Part model, mm, in its own coordinate system. A direction names the side the tool comes from. Coordinates: 2 decimals unless noted, no trailing zeros. Loops run counter-clockwise (first coordinate to the right, second up) from the corner with the lowest first, then second, coordinate; pieces in that order, holes last. Notation, with made-up numbers: (-10.75, 77) - (-0.75, 77) arc R35 ccw to (-0.75, 111) - close; hole circle Ø8 at (-35, 6). An arc over 180 degrees is marked (long way). Answer as CSV lines item,"result".
from build123d import *

# Parameters (mm, degrees)
F0_W          = 200
F0_H          = 200
F1_DEPTH      = 100
F1_DEPTH_BACK = 100
F2_R          = 12.7
F3_R          = 25
F4_DEPTH      = 12.7
F5_R          = 25
F6_DEPTH      = 12.7
F7_R          = 25
F9_DEPTH      = 12.7
F10_R         = 25
F11_DEPTH     = 12.7
F12_R         = 25
F13_DEPTH     = 12.7
F14_R         = 25
F15_DEPTH     = 12.7


with BuildPart() as f1:
    # F0 (on Top) → F1 (new body, two sides)
    with BuildSketch(Plane.XY) as f1_sk:
        Rectangle(F0_W, F0_H)
    extrude(amount=F1_DEPTH)
    extrude(f1_sk.sketch, amount=-F1_DEPTH_BACK)

    # F2
    f2_edges = [f1.edges().sort_by_distance(p)[0] for p in [
        (100, 0, 100),
        (0, 100, 100),
        (-100, 0, 100),
        (0, -100, 100),
        (-100, -100, 0),
        (-100, 0, -100),
        (-100, 100, 0),
        (100, 0, -100),
        (0, 100, -100),
        (0, -100, -100),
        (100, 100, 0),
        (100, -100, 0),
    ]]
    fillet(f2_edges, radius=F2_R)

    # F3 (on face) → F4 (cut)
    with BuildSketch(Plane.XZ.offset(100)):
        Circle(F3_R)
    extrude(amount=-F4_DEPTH, mode=Mode.SUBTRACT)

    # F5 (on face) → F6 (cut)
    with BuildSketch(Plane(origin=(0, 100, 0), x_dir=(-1, 0, 0), z_dir=(0, 1, 0))):
        with Locations((-49.8331896961, 49.8331896961)):
            Circle(F5_R)
        with Locations((3.5068103039, 49.8331896961)):
            Circle(F5_R)
        with Locations((56.8468103039, 49.8331896961)):
            Circle(F5_R)
        with Locations((-49.8331896961, -49.2268103039)):
            Circle(F5_R)
        with Locations((3.5068103039, -49.2268103039)):
            Circle(F5_R)
        with Locations((56.8468103039, -49.2268103039)):
            Circle(F5_R)
    extrude(amount=-F6_DEPTH, mode=Mode.SUBTRACT)

    # F7 (on face) → F9 (cut)
    with BuildSketch(Plane(origin=(-100, 0, 0), x_dir=(0, -1, 0), z_dir=(-1, 0, 0))):
        with Locations((-43.65, 43.65)):
            Circle(F7_R)
        with BuildLine():
            ThreePointArc((24.561363538, -59.7938520193), (52.2460481749, -67.1256886113), (68.65, -43.65))
            ThreePointArc((68.65, -43.65), (67.1342312954, -35.077317779), (62.770729563, -27.5441718319))
            ThreePointArc((62.770729563, -27.5441718319), (27.5572450229, -24.5833313789), (24.561363538, -59.7938520193))
        make_face()
        with BuildLine():
            ThreePointArc((62.770729563, -27.5441718319), (67.1342312954, -35.077317779), (68.65, -43.65))
            ThreePointArc((68.65, -43.65), (52.2460481749, -67.1256886113), (24.561363538, -59.7938520193))
            ThreePointArc((24.561363538, -59.7938520193), (52.254775322, -67.1722551466), (68.6820931009, -43.6880238512))
            ThreePointArc((68.6820931009, -43.6880238512), (67.1577817122, -35.0919756763), (62.770729563, -27.5441718319))
        make_face()
        with BuildLine():
            ThreePointArc((24.561363538, -59.7938520193), (27.5572450229, -24.5833313789), (62.770729563, -27.5441718319))
            ThreePointArc((62.770729563, -27.5441718319), (27.525151922, -24.5453075277), (24.561363538, -59.7938520193))
        make_face()
        with Locations((-43.688, -44.704)):
            Circle(F7_R)
        with Locations((43.7200931009, 44.6659761488)):
            Circle(F7_R)
        Circle(F7_R)
    extrude(amount=-F9_DEPTH, mode=Mode.SUBTRACT)

    # F10 (on face) → F11 (cut)
    with BuildSketch(Plane(origin=(0, 0, -100), x_dir=(1, 0, 0), z_dir=(0, 0, -1))):
        with Locations((43.65, 43.65)):
            Circle(F10_R)
        Circle(F10_R)
        with Locations((-43.65, -43.65)):
            Circle(F10_R)
    extrude(amount=-F11_DEPTH, mode=Mode.SUBTRACT)

    # F12 (on face) → F13 (cut)
    with BuildSketch(Plane.XY.offset(100)):
        with Locations((-43.65, 43.65)):
            Circle(F12_R)
        with Locations((43.65, 43.65)):
            Circle(F12_R)
        with Locations((43.65, -43.65)):
            Circle(F12_R)
        with Locations((-43.65, -43.65)):
            Circle(F12_R)
    extrude(amount=-F13_DEPTH, mode=Mode.SUBTRACT)

    # F14 (on face) → F15 (cut)
    with BuildSketch(Plane.YZ.offset(100)):
        with Locations((-43.65, 43.65)):
            Circle(F14_R)
        with Locations((43.65, -43.65)):
            Circle(F14_R)
    extrude(amount=-F15_DEPTH, mode=Mode.SUBTRACT)


solid = f1.part
Q1. Which spindle directions (+Z, -Z, +X, -X, +Y, -Y) get a long thin tool onto all of the face, cutting with end or side? Do faces 1 (the face through (43, 44, 87.3)), 2 (the face through (-51.427, 93.739, 25.428)), 3 (the face through (-93.74, -38.3, 20.26)), 4 (the face through (18, -18, -100)), 5 (the face through (57.09, -64.73, -93.74)). Say none if no direction does.
Results:
face 1,"+Z"
face 2,"+Y"
face 3,"-X"
face 4,"-Z, +X, -X, +Y, -Y"
face 5,"-Z"
Q2. Saw through at A-A (y = 0). Give the cut face in (x, z).
Results:
outline,"(-100, -87.3) arc R12.7 ccw to (-87.3, -100) - (-25, -100) - (-25, -87.3) - (25, -87.3) - (25, -100) - (87.3, -100) arc R12.7 ccw to (100, -87.3) - (100, 87.3) arc R12.7 ccw to (87.3, 100) - (-87.3, 100) arc R12.7 ccw to (-100, 87.3) - (-100, 25) - (-87.3, 25) - (-87.3, -25) - (-100, -25) - close"
Q3. Saw through at C-C (x = 43.65). Give the cut face in (y, z).
Results:
outline,"(-100, -87.3) arc R12.7 ccw to (-87.3, -100) - (-68.65, -100) - (-68.65, -87.3) - (-18.65, -87.3) - (-18.65, -100) - (87.3, -100) arc R12.7 ccw to (100, -87.3) - (100, -73.45) - (87.3, -73.45) - (87.3, -25) - (100, -25) - (100, 25.61) - (87.3, 25.61) - (87.3, 74.06) - (100, 74.06) - (100, 87.3) arc R12.7 ccw to (87.3, 100) - (68.65, 100) - (68.65, 87.3) - (18.65, 87.3) - (18.65, 100) - (-18.65, 100) - (-18.65, 87.3) - (-68.65, 87.3) - (-68.65, 100) - (-87.3, 100) arc R12.7 ccw to (-100, 87.3) - close"
Q4. Wall check: L1, parallel to Z at x = -90, y = 43.65; L2, parallel to X at y = -43, z = 90; L3, parallel to Z at x = 0, y = -94.5. Give the ranges that are in metal, low to high.
Results:
L1,"z = -99.71 to -69.7, -19.7 to 18.65, 68.65 to 99.71"
L2,"x = -99.71 to -68.64, -18.66 to 18.66, 68.64 to 99.71"
L3,"z = -97.76 to -25, 25 to 97.76"
Q5. Two-plate mould, pull along Z, no slides. Class faces 6 (the face through (87.3, 43, -43)), 7 (the face through (1.22, -96.18, -96.38)), 8 (the face through (-96.38, -96.18, 1.22)): released by +Z, released by -Z, zero draft, split by the parting line, or undercut.
Results:
face 6,"undercut"
face 7,"released by -Z"
face 8,"zero draft"
Q6. Flat gauge pins, fed straight in: pin 1 (1.5 mm diameter, centred on x = 42, y = 42, fed in from +Z); pin 2 (15 mm diameter, centred on y = 53, z = -50.5, fed in from -X); pin 3 (5 mm diameter, centred on x = -14.5, z = 36, fed in from +Y). Where does each tip first touch, or does it go through?
Results:
pin 1,"stops at z = 87.3"
pin 2,"stops at x = -87.3"
pin 3,"stops at y = 87.3"
